Build history of the part. All positions in model axes, mm. Round coordinates to 2 decimals unless told otherwise and drop trailing zeros. Loops run counter-clockwise (first coordinate to the right, second up) from the corner with the lowest first, then second, coordinate; pieces in that order, holes last. Notation, with made-up numbers: M -40,71 L 2,71 A27 cw 2,93 Z; hole C 39,-0.5 d5. An arc over 180 degrees is marked long. One line per item, written item: value.
```python
from build123d import *

# Parameters (mm, degrees)
SKETCH_1_R                  = 50
SKETCH_1_R_2                = 24
EXTRUDE_1_DEPTH             = 4
PATTERN_CIRCULAR_1_COUNT    = 6
CHAMFER_1_SIZE              = 2
HOLE_WIZARD_M32_D           = 3.15
PATTERN_LINEAR_1_COUNT      = 2
PATTERN_LINEAR_1_PITCH      = 18
PATTERN_LINEAR_1_COUNT_DIR2 = 2
PATTERN_LINEAR_1_PITCH_DIR2 = 90
HOLE_WIZARD_M52_D           = 5.2
PATTERN_CIRCULAR_3_COUNT    = 2
PATTERN_CIRCULAR_3_ANGLE    = 45
F_3_THE_OTHER_WAY_COUNT     = 2
F_3_THE_OTHER_WAY_ANGLE     = 45


with BuildPart() as part:
    # Эскиз1 → Бобышка-Вытянуть1 (new body)
    with BuildSketch(Plane(origin=(0, 0, 0), x_dir=(1, 0, 0), z_dir=(0, 1, 0))):
        with Locations(Location((0, 0, 0), (0, 0, 270))):
            Circle(SKETCH_1_R)
        with Locations(Location((0, 0, 0), (0, 0, 270))):
            Circle(SKETCH_1_R_2, mode=Mode.SUBTRACT)
    extrude(amount=EXTRUDE_1_DEPTH)

    # Эскиз3 → Сверло под метчик  спиральное M31 (revolve, cut)
    with BuildSketch(Plane(origin=(28.5, 4, 0), x_dir=(0, 0, 1), z_dir=(1, 0, 0))):
        Polygon((0, 0), (0, 8.946355475), (1.575, 8), (1.575, 0), align=None)
    hole_wizard_m31 = revolve(axis=Axis((28.5, 10.35, 0), (0, -1, 0)), mode=Mode.SUBTRACT)

    # Круговой массив1: Сверло под метчик  спиральное M31 ×6 about axis
    pattern_circular_1_axis = Axis((0, 0, 0), (0, 1, 0))
    for i in range(1, PATTERN_CIRCULAR_1_COUNT):
        add(hole_wizard_m31.rotate(pattern_circular_1_axis, i * 360 / PATTERN_CIRCULAR_1_COUNT), mode=Mode.SUBTRACT)

    # Фаска1
    chamfer_1_edges = [part.edges().sort_by_distance(p)[0] for p in [
        (28.5, 0, -1.575),
        (12.886009989, 0, -25.469224008),
        (-15.613990011, 0, -23.894224008),
        (-28.5, 0, 1.575),
        (-12.886009989, 0, 25.469224008),
        (15.613990011, 0, 23.894224008),
    ]]
    chamfer(chamfer_1_edges, length=CHAMFER_1_SIZE)

    # Сверло под метчик  спиральное M32 (through all)
    with Locations(Plane(origin=(0, 0, 0), x_dir=(-1, 0, 0), z_dir=(0, -1, 0))):
        with Locations((-9, -45)):
            hole_wizard_m32 = Hole(HOLE_WIZARD_M32_D / 2)

    # Линейный массив1: Hole Wizard M32 2 × 2
    with Locations(*[(-i * PATTERN_LINEAR_1_PITCH, 0, -j * PATTERN_LINEAR_1_PITCH_DIR2) for i in range(PATTERN_LINEAR_1_COUNT) for j in range(PATTERN_LINEAR_1_COUNT_DIR2) if (i, j) != (0, 0)]):
        add(hole_wizard_m32, mode=Mode.SUBTRACT)

    # Сверло под метчик  спиральное M52 (through all)
    with Locations(Plane(origin=(0, 0, 0), x_dir=(-1, 0, 0), z_dir=(0, -1, 0))):
        with Locations((42, 0), (-42, 0)):
            hole_wizard_m52 = Hole(HOLE_WIZARD_M52_D / 2)

    # Круговой массив3: Сверло под метчик  спиральное M52 ×2 about axis
    pattern_circular_3_axis = Axis((0, 0, 0), (0, 1, 0))
    for i in range(1, PATTERN_CIRCULAR_3_COUNT):
        add(hole_wizard_m52.rotate(pattern_circular_3_axis, i * PATTERN_CIRCULAR_3_ANGLE / (PATTERN_CIRCULAR_3_COUNT - 1)), mode=Mode.SUBTRACT)

    # 3 the other way: Сверло под метчик  спиральное M52 ×2 about axis
    f_3_the_other_way_axis = Axis((0, 0, 0), (0, -1, 0))
    for i in range(1, F_3_THE_OTHER_WAY_COUNT):
        add(hole_wizard_m52.rotate(f_3_the_other_way_axis, i * F_3_THE_OTHER_WAY_ANGLE / (F_3_THE_OTHER_WAY_COUNT - 1)), mode=Mode.SUBTRACT)


solid = part.part
```
Item 1: Slice it at C-C, the plane z = -45. Give the cut face in (x, y) (1 decimal).
Check values:
outline: M -21.8,0 L -10.6,0 L -10.6,4 L -21.8,4 Z; M -7.4,0 L 7.4,0 L 7.4,4 L -7.4,4 Z; M 10.6,0 L 21.8,0 L 21.8,4 L 10.6,4 Z
Item 2: Pull direction Z, two halves, no side cores. Call faces 1 (the face through (12, 4, 22)), 2 (the face through (15.02, 1.97, 47.69)), 3 (the face through (14.723, 3.014, -26.184)): pulls with the +Z half, pulls with the -Z half, needs draft (parallel to the pull), parting line crosses it, or undercut.
Check values:
face 1: needs draft
face 2: parting line crosses it
face 3: undercut
Item 3: Slice it at A-A, the plane z = 0. Give the cut face in (x, y) (3 decimals).
Check values:
outline: M -50,0 L -44.6,0 L -44.6,4 L -50,4 Z; M -39.4,0 L -32.075,0 L -30.075,2 L -30.075,4 L -39.4,4 Z; M -26.925,2 L -24.925,0 L -24,0 L -24,4 L -26.925,4 Z; M 24,0 L 24.925,0 L 26.925,2 L 26.925,4 L 24,4 Z; M 30.075,2 L 32.075,0 L 39.4,0 L 39.4,4 L 30.075,4 Z; M 44.6,0 L 50,0 L 50,4 L 44.6,4 Z
Item 4: Wall check: line 1 along X through (y, z) = (3.3, -31); line 2 along X through (y, z) = (0.75, 31.5); line 3 along Z through (x, y) = (-14.5, 3.1). Give the ranges that are in metal, low to high.
Check values:
line 1: x = -39.23 to -31.95, -27.45 to 27.45, 31.95 to 39.23
line 2: x = -38.83 to -31.57, -27.82 to 27.82, 31.57 to 38.83
line 3: z = -47.85 to -26.24, -23.13 to -19.12, 19.12 to 23.13, 26.24 to 47.85
Item 5: Slice it at D-D, the plane x = 14.25. Give the cut face in (y, z).
Check values:
outline: M 0,-47.93 L 4,-47.93 L 4,-26.26 L 2,-26.26 L 0,-28.26 Z; M 0,-21.11 L 2,-23.11 L 4,-23.11 L 4,-19.31 L 0,-19.31 Z; M 0,19.31 L 4,19.31 L 4,23.11 L 2,23.11 L 0,21.11 Z; M 0,28.26 L 2,26.26 L 4,26.26 L 4,47.93 L 0,47.93 Z
Item 6: Drop flat-ended pins along their axis: P1, Ø3.5, axis at x = 14.25, z = 24.68, coming from the +Y side; P2, Ø2, axis at y = 3.5, z = -17.5, coming from the +X side; P3, Ø1, axis at x = 13, y = 0.5, coming from the +Z side; P4, Ø1.5, axis at x = 34, y = 0.5, coming from the -Z side. Give the stop position or say it passes through.
Check values:
P1: stops at y = 4
P2: stops at x = 47.2
P3: stops at z = 48.41
P4: stops at z = -37.34
Item 7: Slice it at B-B, the plane x = 0. Give the cut face in (y, z).
Check values:
outline: M 0,-50 L 4,-50 L 4,-24 L 0,-24 Z; M 0,24 L 4,24 L 4,50 L 0,50 Z
